from build123d import *

# Parameters (mm, degrees)
BOSS_EXTRUDE1_DEPTH      = 1
BOSS_EXTRUDE1_DEPTH_BACK = 10
SKETCH1_R                = 4
SKETCH1_R_2              = 2.6
SKETCH2_R                = 5.5
BOSS_EXTRUDE2_DEPTH      = 3.2
SKETCH3_R                = 4.05
CUT_EXTRUDE1_DEPTH       = 2.9
SKETCH4_R                = 2.6
CUT_EXTRUDE2_DEPTH       = 17.190738093
SKETCH5_R                = 4.5
CUT_EXTRUDE3_DEPTH       = 0.5
CHAMFER1_SIZE            = 1.732050808
CHAMFER1_SIZE_2          = 3


with BuildPart() as part:
    # Sketch1 → Boss-Extrude1 (new, two sides: drawn at the far end of the back side and taken through both)
    with BuildSketch(Plane.XY.offset(-BOSS_EXTRUDE1_DEPTH_BACK)):
        Circle(SKETCH1_R)
        Circle(SKETCH1_R_2, mode=Mode.SUBTRACT)
    extrude(amount=BOSS_EXTRUDE1_DEPTH + BOSS_EXTRUDE1_DEPTH_BACK)

    # Sketch2 → Boss-Extrude2 (add)
    with BuildSketch(Plane.XY.offset(1)):
        Circle(SKETCH2_R)
    extrude(amount=BOSS_EXTRUDE2_DEPTH)

    # Sketch3 → Cut-Extrude1 (cut)
    with BuildSketch(Plane.XY.offset(4.2)):
        Circle(SKETCH3_R)
    extrude(amount=-CUT_EXTRUDE1_DEPTH, mode=Mode.SUBTRACT)

    # Sketch4 → Cut-Extrude2 (cut, through all)
    with BuildSketch(Plane(origin=(0, 0, -10), x_dir=(-1, 0, 0), z_dir=(0, 0, -1))):
        with Locations(Location((0, 0, 0), (0, 0, 180))):
            Circle(SKETCH4_R)
    extrude(amount=-CUT_EXTRUDE2_DEPTH, mode=Mode.SUBTRACT)

    # Sketch5 → Cut-Extrude3 (cut)
    with BuildSketch(Plane.XY.offset(1.3)):
        Circle(SKETCH5_R)
    extrude(amount=CUT_EXTRUDE3_DEPTH, mode=Mode.SUBTRACT)

    # Chamfer1
    # the kernel refuses this chamfer: 3, 1.732050808 mm, written as the material it adds along each edge
    with BuildSketch(Plane(origin=(0, 0, 1), x_dir=(1, 0, 0), z_dir=(0, -1, 0))) as chamfer1_piece_1_section:
        Polygon((4 + CHAMFER1_SIZE, 0), (4, -CHAMFER1_SIZE_2), (4, 0), align=None)
    chamfer1_piece_1 = revolve(axis=Axis((0, 0, 1), (0, 0, 1)), mode=Mode.PRIVATE)
    chamfer1_piece_1 = chamfer1_piece_1 & Plane(origin=(0, 0, -0.731250221), x_dir=(1, 0, 0), z_dir=(0, 0, -1)) * Cylinder(5.5, 23, mode=Mode.PRIVATE)
    add(chamfer1_piece_1)


solid = part.part
Source: CAD feature listing. Evaluate the final solid. Frame: model axes, mm. A direction names the side the tool comes from. Give positions to 0.01 mm unless a question says otherwise; leave off trailing zeros. Write each loop counter-clockwise with the first axis right and the second up, starting at its lowest first coordinate (ties: lowest second). Pieces come first, ordered by that corner, then holes. Notation, with made-up numbers: M -3.75,-7 L 27.25,-7 A27 cw 27.25,11 Z; hole C 50,-30 d8. An arc over 180 degrees is marked long. Answer as a JSON object with one key per item and string values.
Q1. Cut plane A-A, the plane x = 0. Return the cut outline in (y, z), then the cut area to 3 significant figures.
Geometry check:
{"outline": "M -5.5,0.6 L -4,-2 L -4,-10 L -2.6,-10 L -2.6,1.3 L -4.5,1.3 L -4.5,1.8 L -4.05,1.8 L -4.05,4.2 L -5.5,4.2 Z; M 2.6,-10 L 4,-10 L 4,-2 L 5.5,0.6 L 5.5,4.2 L 4.05,4.2 L 4.05,1.8 L 4.5,1.8 L 4.5,1.3 L 2.6,1.3 Z", "area": "45.6 mm^2"}
Q2. Access query for faces 4 (the face through (-1.19, 5.37, 2.37)), 5 (the face through (-0.59, 4.46, 1.55)). Directions: +Z, -Z, +X, -X, +Y, -Y. A direction counts if a zero-diameter tool reaches every point of the face in a straight line with its end or side. Return the directions, or none.
Geometry check:
{"face 4": "+Z, -Z", "face 5": "none"}
Q3. Mould query, pull axis X, two halves, no side actions, for faces 1 (the face through (-0.878, -3.954, 3.017)), 2 (the face through (-2, -4, 4.2)), 3 (the face through (-0.867, -3.905, -6.056)). Classes: +X half, -X half, draft (parallel to the pull), parting line (faces both ways), or undercut.
Geometry check:
{"face 1": "undercut", "face 2": "draft", "face 3": "parting line"}
Q4. Contact query for flat-ended pins moving along their axis: P1, Ø6, axis at y = 0.5, z = -8, coming from the -X side; P2, Ø4, axis at x = -1.5, z = -8, coming from the +Y side; P3, Ø1, axis at y = -3.5, z = -1, coming from the +X side. Output: stop coordinate, or through.
Geometry check:
{"P1": "stops at x = -4", "P2": "stops at y = 4", "P3": "stops at x = 3.6"}
Q5. Ray query, line 1 along Y through (x, z) = (0, 3.35); line 2 along Y through (x, z) = (0, 1.65); line 3 along X through (y, z) = (0, 1.25). Return the intervals inside material, ascending.
Geometry check:
{"line 1": "y = -5.5 to -4.05, 4.05 to 5.5", "line 2": "y = -5.5 to -4.5, 4.5 to 5.5", "line 3": "x = -5.5 to -2.6, 2.6 to 5.5"}
Q6. Cut plane C-C, the plane z = -1.75. Return the cut outline in (x, y), then the cut area to 3 significant figures.
Geometry check:
{"outline": "C 0,0 d8.29; hole C 0,0 d5.2", "area": "32.7 mm^2"}
